Design review of the part built by this model. Coordinates are the model's own, in mm. A direction names the side the tool comes from. Coordinates: 2 decimals unless noted, no trailing zeros. Loops run counter-clockwise (first coordinate to the right, second up) from the corner with the lowest first, then second, coordinate; pieces in that order, holes last. Notation, with made-up numbers: (40, 28.5) -> (76, 28.5) arc R22 ccw to (76, 45.5) -> close; hole circle Ø6 at (77.5, -26.75). An arc over 180 degrees is marked (long way). Use CSV: the item, a comma, the result in double quotes.
```python
from build123d import *

# Parameters (mm, degrees)
SKETCH_1_W      = 2.85
SKETCH_1_H      = 2.9
SKETCH_1_W_2    = 2.9
SKETCH_1_H_2    = 2.85
EXTRUDE_1_DEPTH = 3
FILLET_1_R      = 1.5


with BuildPart() as part:
    # Эскиз1 → Бобышка-Вытянуть1 (new body)
    with BuildSketch(Plane.XY):
        Polygon((0, 22.067640687), (0, 0), (-22.067640687, 0), align=None)
        with Locations((-11.5, 3.45)):
            Rectangle(SKETCH_1_W, SKETCH_1_H, mode=Mode.SUBTRACT)
        with Locations((-3.45, 11.5)):
            Rectangle(SKETCH_1_W_2, SKETCH_1_H_2, mode=Mode.SUBTRACT)
    extrude(amount=EXTRUDE_1_DEPTH)

    # Скругление1
    fillet_1_edges = [part.edges().sort_by_distance(p)[0] for p in [
        (0, 0, 1.5),
        (-22.067640687, 0, 1.5),
        (0, 22.067640687, 1.5),
    ]]
    fillet(fillet_1_edges, radius=FILLET_1_R)


solid = part.part
```
Item 1: Add section D-D (x = -14.75). Give the boundary of the cut face in (y, z), then the cut area to 3 significant figures.
Checked values:
outline,"(0, 0) -> (7.32, 0) -> (7.32, 3) -> (0, 3) -> close"
area,"22.0 mm^2"
Item 2: Add section C-C (y = 4.5). Give the boundary of the cut face in (x, z) (3 decimals).
Checked values:
outline,"(-17.568, 0) -> (-12.925, 0) -> (-12.925, 3) -> (-17.568, 3) -> close; (-10.075, 0) -> (0, 0) -> (0, 3) -> (-10.075, 3) -> close"
Item 3: Clearance check with flat-ended pins moving along their axes: pin 1 (1.5 mm diameter, centred on y = 3.5, z = 1.5, fed in from -X); pin 2 (0.9 mm diameter, centred on y = 11, z = 1.5, fed in from -X). State where each tip first meets the part, or that it passes through.
Checked values:
pin 1,"x = -19.32"
pin 2,"x = -11.52"
Item 4: Add section A-A (y = 11). Give the boundary of the cut face in (x, z), then the cut area to 3 significant figures.
Checked values:
outline,"(-11.07, 0) -> (-4.9, 0) -> (-4.9, 3) -> (-11.07, 3) -> close; (-2, 0) -> (0, 0) -> (0, 3) -> (-2, 3) -> close"
area,"24.5 mm^2"
Item 5: Add section B-B (z = 2.55). Give the boundary of the cut face in (x, y) (3 decimals), then the cut area to 3 significant figures.
Checked values:
outline,"(-19.507, 2.561) arc R1.5 ccw to (-18.446, 0) -> (-1.5, 0) arc R1.5 ccw to (0, 1.5) -> (0, 18.446) arc R1.5 ccw to (-2.561, 19.507) -> close; hole (-12.925, 2) -> (-10.075, 2) -> (-10.075, 4.9) -> (-12.925, 4.9) -> close; hole (-4.9, 10.075) -> (-2, 10.075) -> (-2, 12.925) -> (-4.9, 12.925) -> close"
area,"221 mm^2"
Item 6: Draft analysis for pull direction X (two halves, no side actions). For faces 3 (the face through (-0.9, 19.82, 1.52)), 4 (the face through (-12, 4.9, 1)), 5 (the face through (-12, 2, 1)), 6 (the face through (-19.84, 0.95, 1.52)), state which applies: pulls with the +X half, pulls with the -X half, needs draft (parallel to the pull), parting line crosses it, or undercut.
Checked values:
face 3,"parting line crosses it"
face 4,"undercut"
face 5,"undercut"
face 6,"pulls with the -X half"
Item 7: To check wall thickness, follow line 1 along Y through (x, z) = (-3.5, 2.35) (3 decimals); line 2 along Y through (x, z) = (-11.5, 1.75); line 3 along X through (y, z) = (12, 2.2). State the ranges of each line that lie inside material, in increasing order.
Checked values:
line 1,"0 to 10.075, 12.925 to 18.568"
line 2,"0 to 2, 4.9 to 10.57"
line 3,"-10.07 to -4.9, -2 to 0"
Item 8: Machinability: for faces 1 (the face through (-12.925, 3, 1)), 2 (the face through (-10, 0, 1)), which of the approach directions +Z, -Z, +X, -X, +Y, -Y give a long, thin tool a straight path to every point of the face, cutting with its end or side? Answer none if there is none.
Checked values:
face 1,"+Z, -Z"
face 2,"+Z, -Z, +X, -X, -Y"
